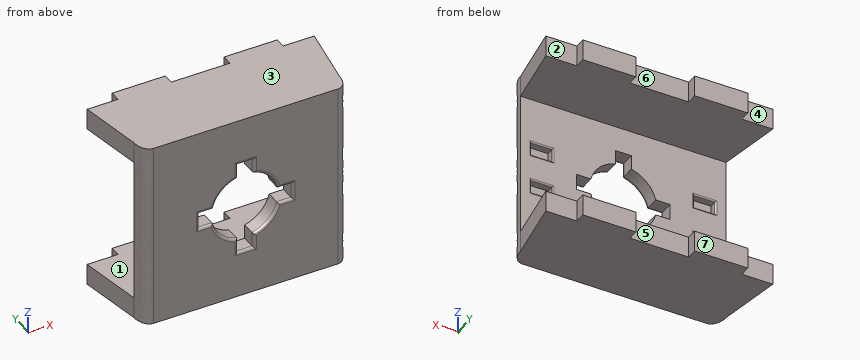
```python
from build123d import *

# Parameters (mm, degrees)
SKETCH1_W             = 19.9
SKETCH1_H             = 7.9
BOSS_EXTRUDE1_DEPTH   = 4
BOSS_EXTRUDE1_2_DEPTH = 4
BOSS_EXTRUDE1_3_DEPTH = 4
BOSS_EXTRUDE1_4_DEPTH = 4
SKETCH2_W             = 85
SKETCH2_H             = 7.9
BOSS_EXTRUDE2_DEPTH   = 24
CHAMFER1_START        = -36
CHAMFER1_DEPTH        = 10
CHAMFER2_SIZE         = 24
CHAMFER2_SIZE_2       = 4
SKETCH4_W             = 77
SKETCH4_H             = 69.8
BOSS_EXTRUDE3_DEPTH   = 6
FILLET1_SIZE          = 6
FILLET1_SIZE_2        = 4
SKETCH7_W             = 8
SKETCH7_H             = 5
CUT_EXTRUDE3_DEPTH    = 65.654930379
SKETCH8_W             = 8
SKETCH8_H             = 20
BOSS_EXTRUDE4_DEPTH   = 3
SKETCH9_R             = 12.5
CUT_EXTRUDE4_DEPTH    = 65.654930379
CUT_EXTRUDE5_DEPTH    = 65.654930379
FILLET2_R             = 1
FILLET3_R             = 0.5


with BuildPart() as part:
    # Sketch1 → Boss-Extrude1 (new body)
    with BuildSketch(Plane(origin=(0, 0, 0), x_dir=(1, 0, 0), z_dir=(0, 1, 0))):
        with Locations((20.95, 30.95)):
            Rectangle(SKETCH1_W, SKETCH1_H)
    extrude(amount=BOSS_EXTRUDE1_DEPTH)



with BuildPart() as body_2:
    # Sketch1 → Boss-Extrude1 2 (new body)
    with BuildSketch(Plane(origin=(0, 0, 0), x_dir=(1, 0, 0), z_dir=(0, 1, 0))):
        with Locations((-20.95, -30.95)):
            Rectangle(SKETCH1_W, SKETCH1_H)
    extrude(amount=BOSS_EXTRUDE1_2_DEPTH)


with BuildPart() as body_3:
    # Sketch1 → Boss-Extrude1 3 (new body)
    with BuildSketch(Plane(origin=(0, 0, 0), x_dir=(1, 0, 0), z_dir=(0, 1, 0))):
        with Locations((20.95, -30.95)):
            Rectangle(SKETCH1_W, SKETCH1_H)
    extrude(amount=BOSS_EXTRUDE1_3_DEPTH)


with BuildPart() as body_4:
    # Sketch1 → Boss-Extrude1 4 (new body)
    with BuildSketch(Plane(origin=(0, 0, 0), x_dir=(1, 0, 0), z_dir=(0, 1, 0))):
        with Locations((-20.95, 30.95)):
            Rectangle(SKETCH1_W, SKETCH1_H)
    extrude(amount=BOSS_EXTRUDE1_4_DEPTH)


with BuildPart() as part_1:
    add(part.part)

    add(body_2.part)  # Boss-Extrude2 merges body 2

    add(body_3.part)  # Boss-Extrude2 merges body 3

    add(body_4.part)  # Boss-Extrude2 merges body 4
    # Sketch2 → Boss-Extrude2 (add)
    with BuildSketch(Plane(origin=(0, 0, 0), x_dir=(1, 0, 0), z_dir=(0, 1, 0))):
        with Locations((0, 30.95)):
            Rectangle(SKETCH2_W, SKETCH2_H)
        with Locations((0, -30.95)):
            Rectangle(SKETCH2_W, SKETCH2_H)
    extrude(amount=-BOSS_EXTRUDE2_DEPTH)

    # Chamfer1: read off the stored shape, not the designer's step
    # Chamfer1 outline → Chamfer1 (cut)
    with BuildSketch(Plane.XY.offset(CHAMFER1_START)):
        Polygon((-42.5, -24), (-38.5, -24), (-42.5, 0), align=None)
        Polygon((42.5, 0), (38.5, -24), (42.5, -24), align=None)
    extrude(amount=CHAMFER1_DEPTH, mode=Mode.SUBTRACT)

    # Chamfer2
    # the kernel refuses this chamfer: 24, 4 mm, written as the material it takes off along each edge
    with BuildSketch(Plane(origin=(42.5, -24, -35.368593459), x_dir=(0, 1, 0), z_dir=(0, 0, 1))) as chamfer2_piece_1:
        Polygon((CHAMFER2_SIZE, 0), (0, CHAMFER2_SIZE_2), (0, 0), align=None)
    extrude(amount=132.637186918, mode=Mode.SUBTRACT)
    with BuildSketch(Plane(origin=(-42.5, -24, 97.268593459), x_dir=(1, 0, 0), z_dir=(0, 0, -1))) as chamfer2_piece_2:
        Polygon((CHAMFER2_SIZE_2, 0), (0, -CHAMFER2_SIZE), (0, 0), align=None)
    extrude(amount=132.637186918, mode=Mode.SUBTRACT)

    # Sketch4 → Boss-Extrude3 (add)
    with BuildSketch(Plane.XZ.offset(24)):
        Rectangle(SKETCH4_W, SKETCH4_H)
    extrude(amount=BOSS_EXTRUDE3_DEPTH)

    # Fillet1
    # a fillet whose section is not a circle: 6, 4 mm, written as the material it takes off along each edge
    with BuildSketch(Plane(origin=(38.5, -30, -49.9), x_dir=(0, 1, 0), z_dir=(0, 0, 1)), Plane(origin=(-38.5, -30, 49.9), x_dir=(0, 1, 0), z_dir=(0, 0, -1))) as fillet1_piece_1:
        with BuildLine():
            Bezier((FILLET1_SIZE, 0), (0, 0), (0, FILLET1_SIZE_2), weights=[1, 0.707106781, 1])
            Line((0, FILLET1_SIZE_2), (0, 0))
            Line((0, 0), (FILLET1_SIZE, 0))
        make_face()
    extrude(amount=99.8, mode=Mode.SUBTRACT)

    # Sketch7 → Cut-Extrude3 (cut, through all)
    with BuildSketch(Plane.XZ.offset(30)):
        with Locations((-30.5, -7.5)):
            Rectangle(SKETCH7_W, SKETCH7_H)
        with Locations((-30.5, 7.5)):
            Rectangle(SKETCH7_W, SKETCH7_H)
        with Locations((30.5, 7.5)):
            Rectangle(SKETCH7_W, SKETCH7_H)
        with Locations((30.5, -7.5)):
            Rectangle(SKETCH7_W, SKETCH7_H)
    extrude(amount=-CUT_EXTRUDE3_DEPTH, mode=Mode.SUBTRACT)

    # Sketch8 → Boss-Extrude4 (add)
    with BuildSketch(Plane.XZ.offset(30)):
        with Locations((-30.5, 0)):
            Rectangle(SKETCH8_W, SKETCH8_H)
        with Locations((30.5, 0)):
            Rectangle(SKETCH8_W, SKETCH8_H)
    extrude(amount=-BOSS_EXTRUDE4_DEPTH)

    # Sketch9 → Cut-Extrude4 (cut, through all)
    with BuildSketch(Plane.XZ.offset(30)):
        with Locations(Location((0, 0, 0), (0, 0, 270))):
            Circle(SKETCH9_R)
    extrude(amount=-CUT_EXTRUDE4_DEPTH, mode=Mode.SUBTRACT)

    # Sketch10 → Cut-Extrude5 (cut, through all)
    with BuildSketch(Plane.XZ.offset(30)):
        Polygon((3, 3), (17.5, 3), (17.5, -3), (3, -3), (3, -17.5), (-3, -17.5), (-3, -3), (-17.5, -3), (-17.5, 3), (-3, 3), (-3, 17.5), (3, 17.5), align=None)
    extrude(amount=-CUT_EXTRUDE5_DEPTH, mode=Mode.SUBTRACT)

    # Fillet2
    fillet2_edges = [part_1.edges().sort_by_distance(p)[0] for p in [
        (8.838834765, -30, -8.838834765),
        (8.838834765, -30, 8.838834765),
        (-8.838834765, -30, 8.838834765),
        (-8.838834765, -30, -8.838834765),
        (-17.5, -30, 0),
        (-14.81733055, -30, -3),
        (0, -30, -17.5),
        (3, -30, -14.81733055),
        (14.81733055, -30, -3),
        (3, -30, 14.81733055),
        (-3, -30, -14.81733055),
        (-14.81733055, -30, 3),
        (-3, -30, 14.81733055),
        (0, -30, 17.5),
        (14.81733055, -30, 3),
        (17.5, -30, 0),
    ]]
    fillet(fillet2_edges, radius=FILLET2_R)

    # Fillet3
    fillet3_edges = [part_1.edges().sort_by_distance(p)[0] for p in [
        (26.5, -24, 7.5),
        (30.5, -24, 5),
        (30.5, -24, 10),
        (34.5, -24, 7.5),
        (26.5, -24, -7.5),
        (30.5, -24, -10),
        (30.5, -24, -5),
        (34.5, -24, -7.5),
        (-30.5, -24, -10),
        (-34.5, -24, -7.5),
        (-30.5, -24, -5),
        (-26.5, -24, -7.5),
        (-26.5, -24, 7.5),
        (-34.5, -24, 7.5),
        (-30.5, -24, 10),
        (-30.5, -24, 5),
    ]]
    fillet(fillet3_edges, radius=FILLET3_R)


solid = part_1.part
```
The model under review builds one solid part; all positions refer to its coordinate system, in mm. Face numbers are marked on the shaded views. A direction names the side the tool comes from. Coordinates: 2 decimals unless noted, no trailing zeros. Write each loop counter-clockwise with the first axis right and the second up, starting at its lowest first coordinate (ties: lowest second). Pieces come first, ordered by that corner, then holes. Notation, with made-up numbers: (56.25, -27.75) - (63.25, -27.75) arc R22 cw to (63.25, -13.75) - close; hole circle Ø9 at (8, 43.25). An arc over 180 degrees is marked (long way). Answer in a Markdown table with one row per item. Add a question column.
Q1. Consider section D-D on y = -12.5. Give the boundary of the cut face in (x, z).
Q2. Clearance check with flat-ended pins moving along their axes: pin 1 (0.8 mm diameter, centred on y = -26, z = -8, fed in from +X); pin 2 (2 mm diameter, centred on y = -25.5, z = 7.5, fed in from +X); pin 3 (1.2 mm diameter, centred on y = 3, z = -29, fed in from +X); pin 4 (8 mm diameter, centred on x = -4, z = -4, fed in from -Y). State where each tip first meets the part, or that it passes through.
Q3. Draft analysis for pull direction X (two halves, no side actions). For the marked faces 6 and 7, state which applies: +X half, -X half, draft (parallel to the pull), parting line (faces both ways), or undercut.
Q4. Consider section B-B on x = 16.5. Give the boundary of the cut face in (y, z), then the cut area to 3 significant figures.
Q5. Consider section A-A on y = -3. Give the boundary of the cut face in (x, z), then the cut area to 3 significant figures.
Q6. Consider section C-C on x = -33. Give the boundary of the cut face in (y, z), then the cut area to 3 significant figures.
Q7. For the marked faces 1, 2, 3, 4 and 5, list the 3-axis set-ups (+Z, -Z, +X, -X, +Y, -Y) from which the entire face can be reached by the end or side of a thin tool; tool diameter is ignored.
Q8. To check wall thickness, follow line 1 along Z through (x, y) = (0, -9); line 2 along Y through (x, z) = (-25, -3.5); line 3 along Y through (x, z) = (-3, -30). State the ranges of each line that lie inside material, in increasing order. Write a range as from..to.
Answers below:
| question | item | result |
|---|---|---|
| 1 | outline | (-40.42, -34.9) - (40.42, -34.9) - (40.42, -27) - (-40.42, -27) - close; (-40.42, 27) - (40.42, 27) - (40.42, 34.9) - (-40.42, 34.9) - close |
| 2 | pin 1 | x = 38.36 |
| 2 | pin 2 | x = 38.49 |
| 2 | pin 3 | x = 30.9 |
| 2 | pin 4 | through |
| 3 | face 6 | undercut |
| 3 | face 7 | draft |
| 4 | outline | (-30, -34.9) - (4, -34.9) - (4, -27) - (-24, -27) - (-24, -3) - (-29, -3) arc R1 ccw to (-30, -4) - close; (-30, 4) arc R1 ccw to (-29, 3) - (-24, 3) - (-24, 27) - (4, 27) - (4, 34.9) - (-30, 34.9) - close |
| 4 | area | 825 mm² |
| 5 | outline | (-42, -34.9) - (42, -34.9) - (42, -27) - (-42, -27) - close; (-42, 27) - (42, 27) - (42, 34.9) - (-42, 34.9) - close |
| 5 | area | 1,330 mm² |
| 6 | outline | (-30, -34.9) - (0, -34.9) - (0, -27) - (-24, -27) - (-24, -10.5) arc R0.5 ccw to (-24.5, -10) - (-27, -10) - (-27, -5) - (-24.5, -5) arc R0.5 ccw to (-24, -4.5) - (-24, 4.5) arc R0.5 ccw to (-24.5, 5) - (-27, 5) - (-27, 10) - (-24.5, 10) arc R0.5 ccw to (-24, 10.5) - (-24, 27) - (0, 27) - (0, 34.9) - (-30, 34.9) - close |
| 6 | area | 768 mm² |
| 7 | face 1 | +X, -X, +Y |
| 7 | face 2 | +Z, -Z, +X, +Y |
| 7 | face 3 | +Z, +X, -X, +Y, -Y |
| 7 | face 4 | +Z, -Z, -X, +Y |
| 7 | face 5 | +Z, -Z, +Y |
| 8 | line 1 | -34.9..-27, 27..34.9 |
| 8 | line 2 | -30..-24 |
| 8 | line 3 | -30..0 |
